```python
from build123d import *

# Parameters (mm, degrees)
SKETCH1_W           = 102
SKETCH1_H           = 129
BOSS_EXTRUDE1_DEPTH = 77
SKETCH2_W           = 122
SKETCH2_H           = 149
BOSS_EXTRUDE2_DEPTH = 3
SKETCH3_W           = 96
SKETCH3_H           = 123
CUT_EXTRUDE1_DEPTH  = 77
SKETCH4_W           = 64
SKETCH4_H           = 89
SKETCH4_W_2         = 62
SKETCH4_H_2         = 34
BOSS_EXTRUDE3_DEPTH = 30
SKETCH5_W           = 60
SKETCH5_H           = 83.431405536
SKETCH5_H_2         = 32
CUT_EXTRUDE2_DEPTH  = 30
FILLET1_R           = 7


with BuildPart() as part:
    # Sketch1 → Boss-Extrude1 (new body)
    with BuildSketch(Plane(origin=(0, 0, 0), x_dir=(1, 0, 0), z_dir=(0, 1, 0))):
        with Locations((51, 64.5)):
            Rectangle(SKETCH1_W, SKETCH1_H)
    extrude(amount=BOSS_EXTRUDE1_DEPTH)

    # Sketch2 → Boss-Extrude2 (add)
    with BuildSketch(Plane(origin=(0, 77, 0), x_dir=(1, 0, 0), z_dir=(0, 1, 0))):
        with Locations((51, 64.5)):
            Rectangle(SKETCH2_W, SKETCH2_H)
    extrude(amount=BOSS_EXTRUDE2_DEPTH)

    # Sketch3 → Cut-Extrude1 (cut)
    with BuildSketch(Plane(origin=(0, 80, 0), x_dir=(1, 0, 0), z_dir=(0, 1, 0))):
        with Locations((51, 64.5)):
            Rectangle(SKETCH3_W, SKETCH3_H)
    extrude(amount=-CUT_EXTRUDE1_DEPTH, mode=Mode.SUBTRACT)

    # Sketch4 → Boss-Extrude3 (add)
    with BuildSketch(Plane(origin=(0, 3, 0), x_dir=(1, 0, 0), z_dir=(0, 1, 0))):
        with Locations((62.459815843, 83.068594464)):
            Rectangle(SKETCH4_W, SKETCH4_H)
        with Locations((34, 20)):
            Rectangle(SKETCH4_W_2, SKETCH4_H_2)
    extrude(amount=BOSS_EXTRUDE3_DEPTH)

    # Sketch5 → Cut-Extrude2 (cut)
    with BuildSketch(Plane(origin=(0, 33, 0), x_dir=(1, 0, 0), z_dir=(0, 1, 0))):
        with Locations((62.459815843, 82.284297232)):
            Rectangle(SKETCH5_W, SKETCH5_H)
        with Locations((33, 19)):
            Rectangle(SKETCH5_W, SKETCH5_H_2)
    extrude(amount=-CUT_EXTRUDE2_DEPTH, mode=Mode.SUBTRACT)

    # Fillet1
    fillet1_edges = [part.edges().sort_by_distance(p)[0] for p in [
        (-10, 78.5, -139),
        (-10, 78.5, 10),
        (112, 78.5, 10),
        (112, 78.5, -139),
    ]]
    fillet(fillet1_edges, radius=FILLET1_R)


solid = part.part
```
Work out the finished part from the listing and answer in its coordinate system (mm). A direction names the side the tool comes from. Round coordinates to 2 decimals unless told otherwise and drop trailing zeros. Write each loop counter-clockwise with the first axis right and the second up, starting at its lowest first coordinate (ties: lowest second). Pieces come first, ordered by that corner, then holes. Notation, with made-up numbers: (-13.75, 64.25) -> (7.25, 64.25) arc R31 ccw to (7.25, 92.25) -> close; hole circle Ø1 at (40, -32.75). An arc over 180 degrees is marked (long way). Write each question's results on one line, items separated by ' | '.
1) Flat-ended cylindrical pins translate along their axes: pin 1 (3 mm diameter, centred on y = 36, z = -64.5, fed in from +X); pin 2 (18 mm diameter, centred on x = 66, z = -91.5, fed in from +Y); pin 3 (12 mm diameter, centred on x = 11, y = 49.5, fed in from +Z). Find the tip coordinate at first contact, or state that the pin passes through.
Findings:
pin 1: stops at x = 102 | pin 2: stops at y = 3 | pin 3: stops at z = 0
2) The part is cut by section C-C (z = -99). Write down the section's boundary in (x, y).
Findings:
outline: (-10, 77) -> (0, 77) -> (0, 0) -> (102, 0) -> (102, 77) -> (112, 77) -> (112, 80) -> (99, 80) -> (99, 3) -> (94.46, 3) -> (94.46, 33) -> (92.46, 33) -> (92.46, 3) -> (32.46, 3) -> (32.46, 33) -> (30.46, 33) -> (30.46, 3) -> (3, 3) -> (3, 80) -> (-10, 80) -> close
3) The part is cut by section A-A (x = 45). Write down the section's boundary in (y, z).
Findings:
outline: (0, -129) -> (77, -129) -> (77, -139) -> (80, -139) -> (80, -126) -> (33, -126) -> (33, -124) -> (3, -124) -> (3, -40.57) -> (33, -40.57) -> (33, -38.57) -> (3, -38.57) -> (3, -37) -> (33, -37) -> (33, -35) -> (3, -35) -> (3, -3) -> (80, -3) -> (80, 10) -> (77, 10) -> (77, 0) -> (0, 0) -> close
4) Which of the six approach directions +Z, -Z, +X, -X, +Y, -Y give full straight-line access (tool end or side, diameter ignored) to faces 5 (the flat face through (102, 38, -64)), 6 (the flat face through (50, 51, -126)), 7 (the flat face through (50, 38, -129))?
Findings:
face 5: +Z, -Z, +X, -Y | face 6: +Y | face 7: -Z, +X, -X, -Y
5) The part is cut by section B-B (y = 68). Write down the section's boundary in (x, z), and give its area (3 significant figures).
Findings:
outline: (0, -129) -> (102, -129) -> (102, 0) -> (0, 0) -> close; hole (3, -126) -> (99, -126) -> (99, -3) -> (3, -3) -> close | area: 1,350 mm²
6) Consider line 1 along Z through (x, y) = (28, 17.5); line 2 along Z through (x, y) = (91.5, 30); line 3 along X through (y, z) = (32, -5.5). Determine where each line is inside the solid, lowest interval first. Write a range as [from, to].
Findings:
line 1: z = [-129, -126], [-37, -35], [-3, 0] | line 2: z = [-129, -124], [-40.57, -38.57], [-3, 0] | line 3: x = [0, 3], [63, 65], [99, 102]
7) For a pull along X with two mould halves and no side action, classify faces 1 (the flat face through (92.46, 18, -82)), 2 (the flat face through (-4, 80, -66)), 3 (the flat face through (99, 42, -64)), 4 (the cylindrical face through (-7.9, 78.5, -137)) as +X half, -X half, draft (parallel to the pull), parting line (faces both ways), or undercut.
Findings:
face 1: undercut | face 2: draft | face 3: undercut | face 4: -X half
8) The part is cut by section D-D (y = 18). Write down the section's boundary in (x, z).
Findings:
outline: (0, -129) -> (102, -129) -> (102, 0) -> (0, 0) -> close; hole (3, -126) -> (30.46, -126) -> (30.46, -38.57) -> (94.46, -38.57) -> (94.46, -126) -> (99, -126) -> (99, -3) -> (65, -3) -> (65, -37) -> (3, -37) -> close; hole (3, -35) -> (63, -35) -> (63, -3) -> (3, -3) -> close; hole (32.46, -124) -> (92.46, -124) -> (92.46, -40.57) -> (32.46, -40.57) -> close
